For this review, use the dimensioned drawing (mm, ordinates from the lowest corner) and the shaded views. A direction names the side the tool comes from. Give positions to 0.01 mm unless a question says otherwise; leave off trailing zeros. Order: outer loops, then holes, each group sorted by start corner. A loop starts at its lowest first (then second) coordinate and runs counter-clockwise, first axis right, second up. Notation, with made-up numbers: (-27, 72) - (7, 72) arc R25 cw to (7, 104) - close; hole circle Ø11 at (51.5, 52). An arc over 180 degrees is marked (long way). Use a Markdown table: item, result. Add a question column.
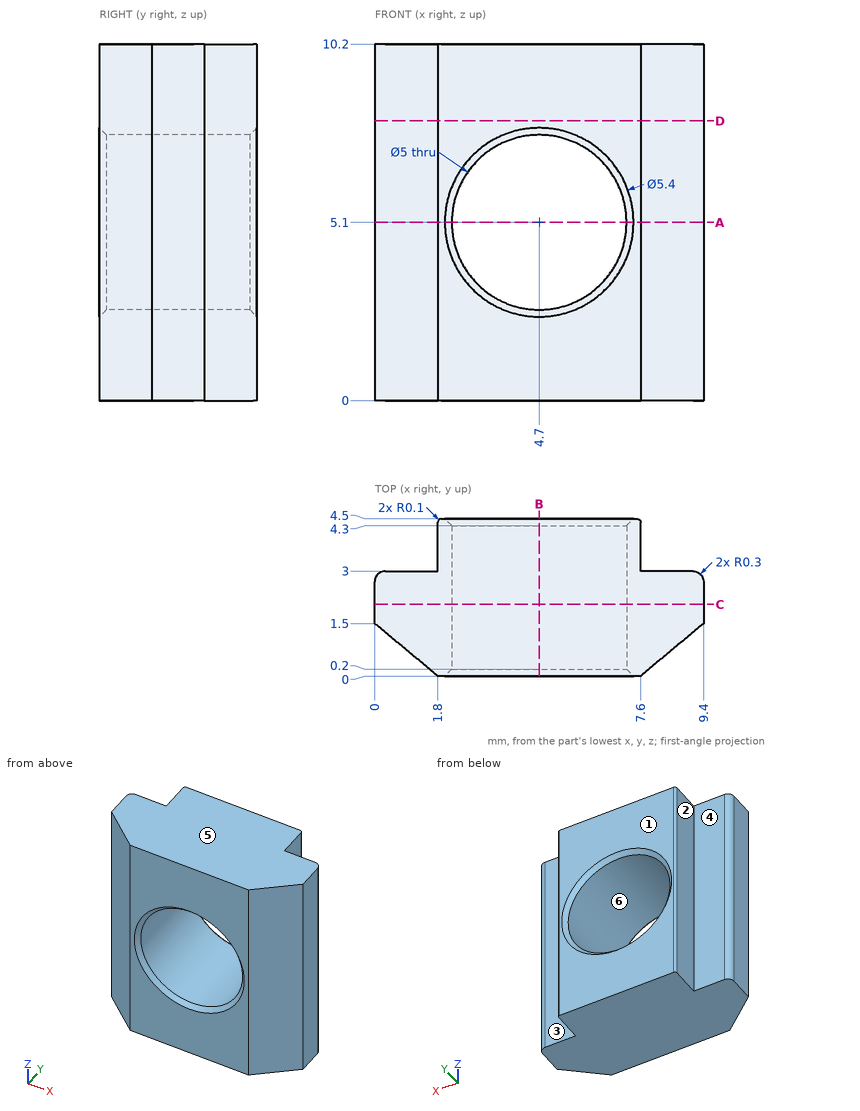
Q1. Machinability: for the marked faces 1, 2 and 3, which of the approach directions +Z, -Z, +X, -X, +Y, -Y give a long, thin tool a straight path to every point of the face, cutting with its end or side? Answer none if there is none.
Q2. Wall thickness on probe 1 along X at (y, z) = (2.4, 5.1); probe 2 along X at (y, z) = (1.4, 7); probe 3 along Z at (x, y) = (4.7, 1.7): over which ranges is each line inside the solid? List them lowest first.
Q3. Clearance check with a flat-ended pin moving along its axis: P1, Ø1.2, axis at x = 8.5, z = 7, coming from the +Y side. State where the tip first meets the part, or that it passes through.
Q4. We need section A-A (z = 5.1). Write out the cut boundary in (x, y).
Q5. We need section D-D (z = 8). Write out the cut boundary in (x, y), plus the area to 3 significant figures.
Q6. Draft analysis for pull direction Z (two halves, no side actions). For the marked faces 4, 5 and 6, state which applies: pulls with the +Z half, pulls with the -Z half, needs draft (parallel to the pull), parting line crosses it, or undercut.
Q7. We need section C-C (y = 2.05). Write out the cut boundary in (x, z).
Q8. We need section B-B (x = 4.7). Write out the cut boundary in (y, z).
Here are the results:
| question | item | result |
|---|---|---|
| 1 | face 1 | +Z, -Z, +X, -X, +Y |
| 1 | face 2 | +Z, -Z, -X, +Y |
| 1 | face 3 | +Z, -Z, +X, +Y |
| 2 | probe 1 | 0 to 2.2, 7.2 to 9.4 |
| 2 | probe 2 | 0.12 to 3.08, 6.32 to 9.28 |
| 2 | probe 3 | 0 to 2.6, 7.6 to 10.2 |
| 3 | P1 | y = 3 |
| 4 | outline | (0, 1.5) - (1.8, 0) - (2, 0) - (2.2, 0.2) - (2.2, 4.3) - (2, 4.5) - (1.9, 4.5) arc R0.1 ccw to (1.8, 4.4) - (1.8, 3) - (0.3, 3) arc R0.3 ccw to (0, 2.7) - close; (7.2, 0.2) - (7.4, 0) - (7.6, 0) - (9.4, 1.5) - (9.4, 2.7) arc R0.3 ccw to (9.1, 3) - (7.6, 3) - (7.6, 4.4) arc R0.1 ccw to (7.5, 4.5) - (7.4, 4.5) - (7.2, 4.3) - close |
| 5 | outline | (0, 1.5) - (1.8, 0) - (7.6, 0) - (9.4, 1.5) - (9.4, 2.7) arc R0.3 ccw to (9.1, 3) - (7.6, 3) - (7.6, 4.4) arc R0.1 ccw to (7.5, 4.5) - (1.9, 4.5) arc R0.1 ccw to (1.8, 4.4) - (1.8, 3) - (0.3, 3) arc R0.3 ccw to (0, 2.7) - close |
| 5 | area | 34.2 mm2 |
| 6 | face 4 | needs draft |
| 6 | face 5 | pulls with the +Z half |
| 6 | face 6 | undercut |
| 7 | outline | (0, 0) - (9.4, 0) - (9.4, 10.2) - (0, 10.2) - close; hole circle Ø5 at (4.7, 5.1) |
| 8 | outline | (0, 0) - (4.5, 0) - (4.5, 2.4) - (4.3, 2.6) - (0.2, 2.6) - (0, 2.4) - close; (0, 7.8) - (0.2, 7.6) - (4.3, 7.6) - (4.5, 7.8) - (4.5, 10.2) - (0, 10.2) - close |
